Work out the finished part from the listing and answer in its coordinate system (mm). Face numbers are marked on the shaded views. A direction names the side the tool comes from. Give positions to 0.01 mm unless a question says otherwise; leave off trailing zeros. Loops run counter-clockwise (first coordinate to the right, second up) from the corner with the lowest first, then second, coordinate; pieces in that order, holes last. Notation, with made-up numbers: M 53.5,34.25 L 65.5,34.25 A7 ccw 65.5,46.25 Z; hole C 18,-33.75 d2. An arc over 180 degrees is marked long. Use a Markdown table: item, result.
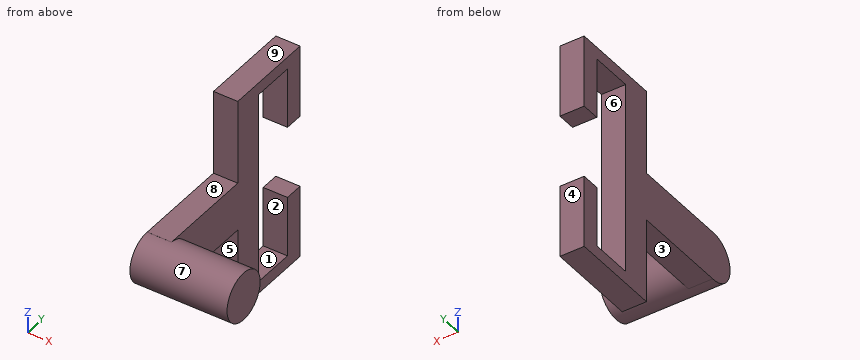
```python
from build123d import *

# Parameters (mm, degrees)
SKETCH2_R           = 12.7
BOSS_EXTRUDE1_DEPTH = 50.8
SKETCH3_W           = 25.4
SKETCH3_H           = 50.8
BOSS_EXTRUDE2_DEPTH = 12.7
SKETCH5_W           = 101.6
SKETCH5_H           = 16.002
BOSS_EXTRUDE3_DEPTH = 12.7
SKETCH6_W           = 6.35
SKETCH6_H           = 38.1
BOSS_EXTRUDE4_DEPTH = 12.7
SKETCH7_W           = 38.1
SKETCH7_H           = 9.652
BOSS_EXTRUDE5_DEPTH = 12.7


with BuildPart() as part:
    # Sketch2 → Boss-Extrude1 (new body)
    with BuildSketch(Plane(origin=(0, 0, 0), x_dir=(0, 0, -1), z_dir=(1, 0, 0))):
        Circle(SKETCH2_R)
    extrude(amount=BOSS_EXTRUDE1_DEPTH)

    # Sketch3 → Boss-Extrude2 (add)
    with BuildSketch(Plane.ZY):
        with Locations((0.014597196, 26.008732875)):
            Rectangle(SKETCH3_W, SKETCH3_H)
    extrude(amount=-BOSS_EXTRUDE2_DEPTH)


with BuildPart() as body_2:
    # Sketch5 → Boss-Extrude3 (new body)
    with BuildSketch(Plane(origin=(0, 0, 0), x_dir=(0, 0, -1), z_dir=(1, 0, 0))):
        with Locations((0, 59.392294155)):
            Rectangle(SKETCH5_W, SKETCH5_H)
    extrude(amount=BOSS_EXTRUDE3_DEPTH)

    # Sketch6 → Boss-Extrude4 (add)
    with BuildSketch(Plane(origin=(0, 0, 0), x_dir=(0, 0, -1), z_dir=(1, 0, 0))):
        with Locations((-53.975, 70.441294155)):
            Rectangle(SKETCH6_W, SKETCH6_H)
        with Locations((53.975, 70.441294155)):
            Rectangle(SKETCH6_W, SKETCH6_H)
    extrude(amount=BOSS_EXTRUDE4_DEPTH)

    # Sketch7 → Boss-Extrude5 (add)
    with BuildSketch(Plane(origin=(0, 0, 0), x_dir=(0, 0, -1), z_dir=(1, 0, 0))):
        with Locations((-38.1, 94.317294155)):
            Rectangle(SKETCH7_W, SKETCH7_H)
        with Locations((38.1, 94.317294155)):
            Rectangle(SKETCH7_W, SKETCH7_H)
    extrude(amount=BOSS_EXTRUDE5_DEPTH)


with BuildPart() as part_1:
    add(part.part)

    # Combine1: union body 2
    add(body_2.part)


solid = part_1.part
```
(1) Consider probe 1 along Y at (x, z) = (11.5, 48); probe 2 along X at (y, z) = (40, -10); probe 3 along Z at (x, y) = (5.5, 17). Determine where each line is inside the solid, lowest interval first. Write a range as [from, to].
Entries:
| item | result |
|---|---|
| probe 1 | y = [51.39, 67.39], [89.49, 99.14] |
| probe 2 | x = [0, 12.7] |
| probe 3 | z = [-12.69, 12.71] |
(2) A cutting plane is placed at A-A (y = 85). Write down the section's boundary in (x, z).
Entries:
| item | result |
|---|---|
| outline | M 0,-57.15 L 12.7,-57.15 L 12.7,-50.8 L 0,-50.8 Z; M 0,50.8 L 12.7,50.8 L 12.7,57.15 L 0,57.15 Z |
(3) A cutting plane is placed at B-B (z = 32.5). Write down the section's boundary in (x, y), and give its area (3 significant figures).
Entries:
| item | result |
|---|---|
| outline | M 0,51.39 L 12.7,51.39 L 12.7,67.39 L 0,67.39 Z; M 0,89.49 L 12.7,89.49 L 12.7,99.14 L 0,99.14 Z |
| area | 326 mm² |
(4) The mould has two halves that part along Z. Classify the marked faces 1, 2, 3 and 4: released by +Z, released by -Z, zero draft, split by the parting line, or undercut.
Entries:
| item | result |
|---|---|
| face 1 | undercut |
| face 2 | undercut |
| face 3 | released by -Z |
| face 4 | zero draft |
(5) A cutting plane is placed at D-D (z = 0). Write down the section's boundary in (x, y).
Entries:
| item | result |
|---|---|
| outline | M 0,-12.7 L 50.8,-12.7 L 50.8,12.7 L 12.7,12.7 L 12.7,67.39 L 0,67.39 Z |
(6) Which of the six approach directions +Z, -Z, +X, -X, +Y, -Y give full straight-line access (tool end or side, diameter ignored) to the marked faces 5, 6, 7, 8 and 9?
Entries:
| item | result |
|---|---|
| face 5 | -Z, +X, -X, -Y |
| face 6 | +X, -X |
| face 7 | +X |
| face 8 | +Z, +X, -X, -Y |
| face 9 | +Z, +X, -X, +Y, -Y |
(7) Given P1, Ø6.5, axis at x = 4, y = 31, coming from the -Z side; P2, Ø4, axis at x = 7.5, z = -43, coming from the -Y side; P3, Ø1, axis at x = 26, z = 10, coming from the -Y side, each flat-ended and moving along its own axis, determine where each tip first touches the part or whether it passes through.
Entries:
| item | result |
|---|---|
| P1 | stops at z = -12.69 |
| P2 | stops at y = 51.39 |
| P3 | stops at y = -8.43 |
